Autodesk Inventor part; units mm, degrees
ref_plane "YZ Plane" through (0, 0, 0) normal (1, 0, 0) x (0, 1, 0)
ref_plane "XZ Plane" through (0, 0, 0) normal (0, 1, 0) x (-1, 0, 0)
ref_plane "XY Plane" through (0, 0, 0) normal (0, 0, 1) x (1, 0, 0)
sketch "main" plane through (0, 0, 0) normal (0, 0, 1) x (1, 0, 0)
  line L0 (-30.6986, 36.9894) -> (-3.5098, -9.6529)
  line L1 (14.2033, 60.1599) -> (14.2442, -4.8501)
  circle A0 centre (4.7192, -4.8561) radius 2.1844
  arc A1 (-3.5098, -9.6529) -> (14.2442, -4.8501) centre (4.7192, -4.8561) ccw
  line L2 (4.7192, -4.8561) -> (42.8192, -4.8561) construction
  circle A2 centre (1.3985, 33.099) radius 2.1844
  line L3 (4.7192, -4.8561) -> (69.8067, -4.8561) construction
  circle A3 centre (7.8533, 60.1559) radius 2.1209
  arc A4 (14.2033, 60.1599) -> (3.0678, 64.3299) centre (7.8533, 60.1559) ccw
  line L4 (1.3985, 33.099) -> (26.7985, 33.099) construction
  circle A5 centre (-22.4696, 41.7863) radius 2.1844
  arc A6 (-23.1365, 51.2879) -> (-30.6986, 36.9894) centre (-22.4696, 41.7863) ccw
  arc A7 (-23.1365, 51.2879) -> (3.0678, 64.3299) centre (-25.8203, 89.5265) ccw
  point P0 (-13.3913, 7.903)
  dimension "d33" = 19.05
  dimension "d41" = 4.3688
  dimension "d48" = 12.7
  dimension "d52" = 19.05
sketch "Sketch1" plane through (0, 0, 0) normal (0, 0, 1) x (1, 0, 0)
  line L0 (-25.5568, 5.0437) -> (1.632, -41.5986)
  line L1 (19.3451, 28.2142) -> (19.386, -36.7958)
  circle A0 centre (9.861, -36.8018) radius 2.1844
  arc A1 (1.632, -41.5986) -> (19.386, -36.7958) centre (9.861, -36.8018) ccw
  line L2 (9.861, -36.8018) -> (47.961, -36.8018) construction
  circle A2 centre (6.5404, 1.1532) radius 2.1844
  line L3 (9.861, -36.8018) -> (74.9485, -36.8018) construction
  circle A3 centre (12.9951, 28.2102) radius 2.1209
  arc A4 (19.3451, 28.2142) -> (8.2097, 32.3842) centre (12.9951, 28.2102) ccw
  line L4 (6.5404, 1.1532) -> (31.9404, 1.1532) construction
  circle A5 centre (-17.3278, 9.8406) radius 2.1844
  arc A6 (-17.9947, 19.3422) -> (-25.5568, 5.0437) centre (-17.3278, 9.8406) ccw
  arc A7 (-17.9947, 19.3422) -> (8.2097, 32.3842) centre (-20.6785, 57.5808) ccw
  point P0 (0, 0)
extrude "Extrusion1" add sketch "Sketch1" along normal blind 1.5875
properties part number "pod_gusset" material "Acetal Resin, White"
The listing builds one solid part. Answer for the finished solid, in the listing's coordinates (mm). Round coordinates to 2 decimals unless told otherwise and drop trailing zeros. Order: outer loops, then holes, each group sorted by start corner. A loop starts at its lowest first (then second) coordinate and runs counter-clockwise, first axis right, second up. Notation, with made-up numbers: (73.25, 18) - (108.25, 18) arc R24 ccw to (108.25, 34) - close; hole circle Ø1 at (13, 73). An arc over 180 degrees is marked (long way). Put each result on its own line as item: value. Start each with the question number.
(1) Determine the mould class of faces 1 (the cylindrical face through (11.31, 29.5, 0.78)), 2 (the flat face through (1, -5, 1.588)), 3 (the cylindrical face through (-3.41, 23.36, 0.78)), 4 (the flat face through (-12.153, -17.951, 0.783)) for opening direction Y: released by +Y, released by -Y, zero draft, split by the parting line, or undercut.
(2) Find section B-B (z = 0.9). Give the vertices of the cut face in (x, y) (3 decimals).
(3) Find section D-D (x = -12.5). Give the vertices of the cut face in (y, z), plus the area to 3 significant figures.
(4) Find section C-C (y = -3.5). Give the vertices of the cut face in (x, z).
(5) Find section A-A (y = 27). Give the vertices of the cut face in (x, z), plus the area to 3 significant figures.
(6) Straight lines are drawn through the part: probe 1 along X at (y, z) = (-37, 0.35); probe 2 along X at (y, z) = (-38.5, 0.45); probe 3 along Y at (x, z) = (-15.5, 0.65). For each, find the intervals that lie inside material, in ascending order. Write a range as from..to.
Reply:
1. face 1: undercut
1. face 2: zero draft
1. face 3: released by +Y
1. face 4: released by -Y
2. outline: (-25.557, 5.044) - (1.632, -41.599) arc R9.525 ccw to (19.386, -36.796) - (19.345, 28.214) arc R6.35 ccw to (8.21, 32.384) arc R38.333 cw to (-17.995, 19.342) arc R9.525 ccw to start; hole circle Ø4.369 at (-17.328, 9.841); hole circle Ø4.369 at (6.54, 1.153); hole circle Ø4.369 at (9.861, -36.802); hole circle Ø4.242 at (12.995, 28.21)
3. outline: (-17.36, 0) - (20.13, 0) - (20.13, 1.59) - (-17.36, 1.59) - close
3. area: 59.5 mm^2
4. outline: (-20.58, 0) - (19.37, 0) - (19.37, 1.59) - (-20.58, 1.59) - close
5. outline: (2.43, 0) - (11.25, 0) - (11.25, 1.59) - (2.43, 1.59) - close; (14.74, 0) - (19.35, 0) - (19.35, 1.59) - (14.74, 1.59) - close
5. area: 21.3 mm^2
6. probe 1: -1.05..7.69, 12.04..19.38
6. probe 2: -0.17..8.49, 11.23..19.23
6. probe 3: -12.21..8.64, 11.04..19.6
